The listing builds one solid part. Answer for the finished solid, in the listing's coordinates (mm). Round coordinates to 2 decimals unless told otherwise and drop trailing zeros. Write each loop counter-clockwise with the first axis right and the second up, starting at its lowest first coordinate (ties: lowest second). Pieces come first, ordered by that corner, then holes. Notation, with made-up numbers: (-11.5, -35.5) - (-0.5, -35.5) arc R37 ccw to (-0.5, 2.5) - close; hole circle Ø10 at (-10.5, 20.5). An arc over 180 degrees is marked (long way). Answer as CSV lines item,"result". Start each with the question number.
Item 1: A flat-ended cylindrical pin translates along its axis: pin 1 (1.1 mm diameter, centred on y = 0.5, z = 29.5, fed in from -X). Find the tip coordinate at first contact, or state that the pin passes through.
Item 2: A cutting plane is placed at B-B on z = 19.05. Determine the outline of the cut face in (x, y), and give its area (3 significant figures).
Item 3: A cutting plane is placed at A-A on x = 0. Determine the outline of the cut face in (y, z).
Item 4: A cutting plane is placed at D-D on y = -0.1. State how many separate pieces and enclosed holes the cut face has, and give its area (3 significant figures).
Item 5: Straight lines are drawn through the part: line 1 along X through (y, z) = (0.3, 19.05); line 2 along Z through (x, y) = (32, -0.35); line 3 along X through (y, z) = (-0.55, 40). For each, find the intervals that lie inside material, in ascending order. Write a range as [from, to].
Item 6: A cutting plane is placed at C-C on x = -31.75. Determine the outline of the cut face in (y, z), and give its area (3 significant figures).
```python
from build123d import *

# Parameters (mm, degrees)
BOSS_EXTRUDE1_DEPTH = 1.143
SKETCH2_R           = 2.5527
CUT_EXTRUDE1_DEPTH  = 75.088364782
FILLET1_R           = 3.175


with BuildPart() as part:
    # Sketch1 → Boss-Extrude1 (new, symmetric)
    with BuildSketch(Plane(origin=(0, 0, 0), x_dir=(1, 0, 0), z_dir=(0, 1, 0))):
        Polygon((12.7, -12.7), (38.1, -12.7), (38.1, 12.7), (-38.1, 12.7), (-38.1, -12.7), (-12.7, -12.7), (-12.7, -63.5), (12.7, -63.5), align=None)
    extrude(amount=BOSS_EXTRUDE1_DEPTH, both=True)

    # Sketch2 → Cut-Extrude1 (cut, through all)
    with BuildSketch(Plane(origin=(0, 1.143, 0), x_dir=(1, 0, 0), z_dir=(0, 1, 0))):
        with Locations(Location((-31.75, 0, 0), (0, 0, 270))):
            Circle(SKETCH2_R)
        with Locations(Location((-19.05, 0, 0), (0, 0, 270))):
            Circle(SKETCH2_R)
        with Locations(Location((-6.35, 0, 0), (0, 0, 270))):
            Circle(SKETCH2_R)
        with Locations(Location((6.35, 0, 0), (0, 0, 270))):
            Circle(SKETCH2_R)
        with Locations(Location((19.05, 0, 0), (0, 0, 270))):
            Circle(SKETCH2_R)
        with Locations(Location((0, -57.15, 0), (0, 0, 270))):
            Circle(SKETCH2_R)
        with Locations(Location((31.75, 0, 0), (0, 0, 270))):
            Circle(SKETCH2_R)
        with Locations(Location((0, -44.45, 0), (0, 0, 270))):
            Circle(SKETCH2_R)
        with Locations(Location((0, -31.75, 0), (0, 0, 270))):
            Circle(SKETCH2_R)
        with Locations(Location((0, -19.05, 0), (0, 0, 270))):
            Circle(SKETCH2_R)
    extrude(amount=-CUT_EXTRUDE1_DEPTH, mode=Mode.SUBTRACT)

    # Fillet1
    fillet1_edges = [part.edges().sort_by_distance(p)[0] for p in [
        (38.1, 0, 12.7),
        (12.7, 0, 12.7),
        (12.7, 0, 63.5),
        (-12.7, 0, 63.5),
        (-12.7, 0, 12.7),
        (-38.1, 0, 12.7),
        (-38.1, 0, -12.7),
        (38.1, 0, -12.7),
    ]]
    fillet(fillet1_edges, radius=FILLET1_R)


solid = part.part
```
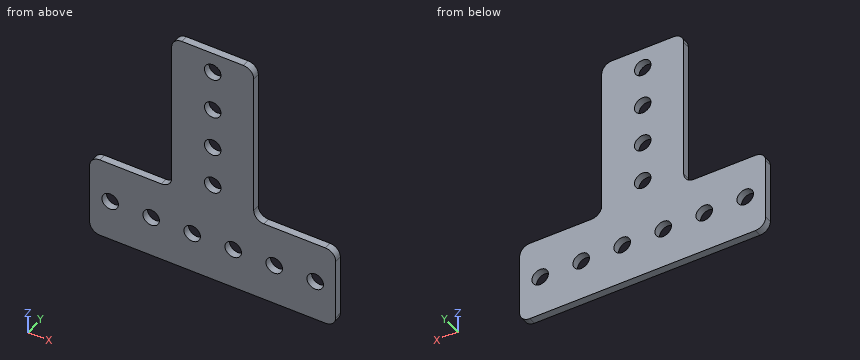
Geometry says:
1,pin 1,"stops at x = -12.7"
2,outline,"(-12.7, -1.14) - (-2.55, -1.14) - (-2.55, 1.14) - (-12.7, 1.14) - close; (2.55, -1.14) - (12.7, -1.14) - (12.7, 1.14) - (2.55, 1.14) - close"
2,area,"46.4 mm^2"
3,outline,"(-1.14, -12.7) - (1.14, -12.7) - (1.14, 16.5) - (-1.14, 16.5) - close; (-1.14, 21.6) - (1.14, 21.6) - (1.14, 29.2) - (-1.14, 29.2) - close; (-1.14, 34.3) - (1.14, 34.3) - (1.14, 41.9) - (-1.14, 41.9) - close; (-1.14, 47) - (1.14, 47) - (1.14, 54.6) - (-1.14, 54.6) - close; (-1.14, 59.7) - (1.14, 59.7) - (1.14, 63.5) - (-1.14, 63.5) - close"
4,separate pieces,"1"
4,enclosed holes,"10"
4,area,"3,010 mm^2"
5,line 1,"x = [-12.7, -2.55], [2.55, 12.7]"
5,line 2,"z = [-12.7, -2.54], [2.54, 12.7]"
5,line 3,"x = [-12.7, 12.7]"
6,outline,"(-1.14, -12.7) - (1.14, -12.7) - (1.14, -2.55) - (-1.14, -2.55) - close; (-1.14, 2.55) - (1.14, 2.55) - (1.14, 12.7) - (-1.14, 12.7) - close"
6,area,"46.4 mm^2"
